Check sheet for the modelled part. Datum: model origin and axes. Units: mm. Face numbers are marked on the shaded views. A direction names the side the tool comes from. Give positions to 0.01 mm unless a question says otherwise; leave off trailing zeros. Write each loop counter-clockwise with the first axis right and the second up, starting at its lowest first coordinate (ties: lowest second). Pieces come first, ordered by that corner, then holes. Notation, with made-up numbers: (29.5, -31.75) -> (62.5, -31.75) arc R18 cw to (62.5, -1.75) -> close; hole circle Ø8 at (12, -15.75). An arc over 180 degrees is marked (long way). Answer as a JSON object with one key per item and string values.
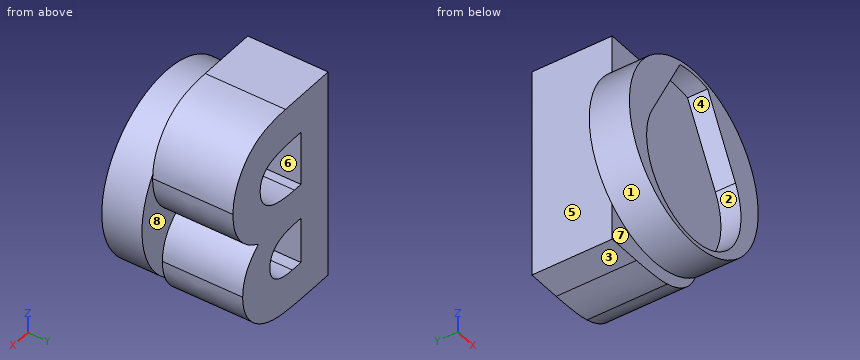
from build123d import *

# Parameters (mm, degrees)
SKETCH1_R           = 22.5
BOSS_EXTRUDE1_DEPTH = 10
BOSS_EXTRUDE2_DEPTH = 20
SKETCH3_R           = 16.5
CUT_EXTRUDE2_DEPTH  = 5


with BuildPart() as part:
    # Sketch1 → Boss-Extrude1 (new body)
    with BuildSketch(Plane(origin=(0, 0, 0), x_dir=(1, 0, 0), z_dir=(0, 1, 0))):
        with Locations(Location((0, 0, 0), (0, 0, 270))):
            Circle(SKETCH1_R)
    extrude(amount=BOSS_EXTRUDE1_DEPTH)

    # Sketch2 → Boss-Extrude2 (add)
    with BuildSketch(Plane(origin=(0, 10, 0), x_dir=(1, 0, 0), z_dir=(0, 1, 0))):
        with BuildLine():
            Line((-14.488149335, -26.70508671), (-14.488149335, 26.211579956))
            Line((-14.488149335, 26.211579956), (-6.007914293, 26.211579956))
            add(Edge.make_bspline(
                [(-6.007914293, 26.211579956), (-5.414244815, 26.211647709), (-4.265505631, 26.211778808), (-2.608174782, 26.15357879), (-1.071140386, 26.078290547), (0.340706119, 25.99406051), (1.629767793, 25.848915327), (2.794084408, 25.69594816), (3.835982274, 25.511479183), (4.480131109, 25.346004797), (4.783184799, 25.268153808)],
                knots=[0, 0, 0, 0, 1.311965854, 2.538629056, 3.664479157, 4.713267157, 5.663616078, 6.530575999, 7.308677837, 8, 8, 8, 8], degree=3))
            add(Edge.make_bspline(
                [(4.783184799, 25.268153808), (5.181125063, 25.158343602), (5.962011612, 24.942860725), (7.080490347, 24.507683744), (8.141523447, 24.023953675), (9.143815418, 23.472108139), (10.08121179, 22.845484813), (10.950150136, 22.139110625), (11.769371306, 21.381339407), (12.509786627, 20.551052288), (13.179000085, 19.673700144), (13.760426595, 18.749512867), (14.265611712, 17.792621882), (14.669892129, 16.790985354), (14.974509828, 15.749216088), (15.197305942, 14.671762602), (15.341707994, 13.555215567), (15.355352093, 12.795592125), (15.362278015, 12.409997424)],
                knots=[0, 0, 0, 0, 1.099996261, 2.158545794, 3.195537121, 4.207578794, 5.205712374, 6.197378256, 7.190519799, 8.17788031, 9.159561366, 10.129234751, 11.085776129, 12.040971148, 13.00380137, 13.975669004, 14.972423361, 16, 16, 16, 16], degree=3))
            add(Edge.make_bspline(
                [(15.362278015, 12.409997424), (15.344168787, 11.914609447), (15.308522997, 10.939499081), (15.080815259, 9.507238371), (14.653827774, 8.153546136), (14.095125035, 6.85347434), (13.335463983, 5.611872259), (12.370841368, 4.429330241), (11.216880916, 3.269436044), (10.331729546, 2.574157712), (9.871325825, 2.212514786)],
                knots=[0, 0, 0, 0, 0.986156485, 1.941127874, 2.875419072, 3.804401753, 4.751181392, 5.761612777, 6.835722519, 8, 8, 8, 8], degree=3))
            add(Edge.make_bspline(
                [(9.871325825, 2.212514786), (10.244414913, 2.022056041), (10.975939394, 1.648619138), (12.014489248, 1.034800345), (12.976073045, 0.381926211), (13.865002238, -0.296867174), (14.662630517, -1.030354847), (15.401893295, -1.77627224), (16.046319182, -2.577357317), (16.622584233, -3.40505788), (17.123464449, -4.271359131), (17.559675885, -5.174798081), (17.928128038, -6.118461074), (18.240142851, -7.09754563), (18.472843581, -8.115419342), (18.624569406, -9.172446243), (18.740740181, -10.265021335), (18.749777175, -11.009256203), (18.754372032, -11.387662164)],
                knots=[0, 0, 0, 0, 1.164658916, 2.283573913, 3.35186032, 4.395461096, 5.390182219, 6.362969632, 7.312859996, 8.245001507, 9.165155236, 10.092416118, 11.032087915, 11.979892451, 12.947605196, 13.931445124, 14.948243989, 16, 16, 16, 16], degree=3))
            add(Edge.make_bspline(
                [(18.754372032, -11.387662164), (18.724554483, -12.110395914), (18.665709669, -13.536708072), (18.235465105, -15.630861893), (17.48955774, -17.616309656), (16.487957959, -19.48516034), (15.25379432, -21.183313786), (13.834860053, -22.670881463), (12.245440572, -23.930074476), (10.779008994, -24.779932076), (9.510661162, -25.350265997), (8.46011235, -25.702882393), (7.331845194, -26.029545689), (6.105192549, -26.258935401), (4.802391955, -26.468898089), (3.410741024, -26.598533402), (1.932840727, -26.686384059), (0.917754918, -26.698726455), (0.394663165, -26.70508671)],
                knots=[0, 0, 0, 0, 1.284142165, 2.534249414, 3.780121997, 5.041676246, 6.291546858, 7.49970053, 8.684500223, 9.883330709, 10.50184324, 11.153274765, 11.851151195, 12.587658647, 13.369265475, 14.195992086, 15.070362669, 16, 16, 16, 16], degree=3))
            Line((0.394663165, -26.70508671), (-14.488149335, -26.70508671))
        make_face()
        with BuildLine():
            Line((-4.990286087, 16.713716709), (-4.990286087, 5.180597051))
            Line((-4.990286087, 5.180597051), (-2.467416162, 5.180597051))
            add(Edge.make_bspline(
                [(-2.467416162, 5.180597051), (-2.124535473, 5.1835871), (-1.462625052, 5.189359209), (-0.50656566, 5.263701973), (0.382415177, 5.390535346), (1.200945746, 5.567499807), (1.956650957, 5.79221887), (2.644703146, 6.062604299), (3.262077073, 6.392503912), (3.979322786, 6.883903943), (4.737503228, 7.607021089), (5.404920943, 8.65171363), (5.798025521, 9.853106078), (5.841806769, 10.700421057), (5.864414767, 11.137962168)],
                knots=[0, 0, 0, 0, 1.065314748, 2.056525647, 2.977365736, 3.853934255, 4.656397591, 5.425096493, 6.14721249, 6.826394842, 8.123232004, 9.372140726, 10.643011755, 12, 12, 12, 12], degree=3))
            add(Edge.make_bspline(
                [(5.864414767, 11.137962168), (5.84632423, 11.547792116), (5.811346902, 12.340181849), (5.415541135, 13.452767604), (4.800776528, 14.438746288), (4.074960502, 15.113568064), (3.391463676, 15.574451442), (2.80621175, 15.87792352), (2.163853815, 16.149588622), (1.451954509, 16.357310381), (0.674579167, 16.513177474), (-0.164496065, 16.627643188), (-1.06671888, 16.705553423), (-1.689886099, 16.710937246), (-2.011603529, 16.713716709)],
                knots=[0, 0, 0, 0, 1.347982417, 2.606269829, 3.849316587, 5.153353503, 5.842674298, 6.568177932, 7.326619318, 8.142485038, 9.012069166, 9.942760135, 10.937925643, 12, 12, 12, 12], degree=3))
            Line((-2.011603529, 16.713716709), (-4.990286087, 16.713716709))
        make_face(mode=Mode.SUBTRACT)
        with BuildLine():
            Line((-4.990286087, -3.638847394), (-4.990286087, -17.207223462))
            Line((-4.990286087, -17.207223462), (-2.255410286, -17.207223462))
            add(Edge.make_bspline(
                [(-2.255410286, -17.207223462), (-1.714721858, -17.204134529), (-0.675180886, -17.198195671), (0.813959715, -17.126440131), (2.167960807, -16.997113416), (3.383234797, -16.835659429), (4.461643108, -16.61691453), (5.399540462, -16.338808424), (6.209788904, -16.032843269), (6.887530146, -15.654939974), (7.441205914, -15.215154252), (7.940840245, -14.76568268), (8.348210945, -14.247174757), (8.670530245, -13.681888592), (8.94949703, -13.0838663), (9.117750095, -12.429755326), (9.245852073, -11.738941952), (9.252901868, -11.26112128), (9.256508784, -11.016651881)],
                knots=[0, 0, 0, 0, 1.753078804, 3.370512758, 4.83203934, 6.162291463, 7.344201807, 8.395507345, 9.331626367, 10.147333109, 10.898971645, 11.62040215, 12.321813352, 13.025280112, 13.727906689, 14.453419512, 15.208716525, 16, 16, 16, 16], degree=3))
            add(Edge.make_bspline(
                [(9.256508784, -11.016651881), (9.248554499, -10.737097279), (9.233061691, -10.192600118), (9.106531742, -9.396759406), (8.876585491, -8.653789298), (8.58695697, -7.944691045), (8.183923494, -7.294852835), (7.704931981, -6.681786232), (7.126187955, -6.126251562), (6.475356533, -5.594648013), (5.716226117, -5.129200305), (4.848440543, -4.725341973), (3.867285527, -4.388054368), (2.769721839, -4.119505755), (1.560561113, -3.891592259), (0.230977803, -3.755502742), (-1.207954859, -3.654286988), (-2.205734185, -3.644110867), (-2.721823214, -3.638847394)],
                knots=[0, 0, 0, 0, 0.845221588, 1.646264278, 2.427170338, 3.19324141, 3.95557735, 4.731569926, 5.540061037, 6.376114724, 7.268642756, 8.224665384, 9.265483498, 10.400594375, 11.639216012, 12.983232105, 14.439614077, 16, 16, 16, 16], degree=3))
            Line((-2.721823214, -3.638847394), (-4.990286087, -3.638847394))
        make_face(mode=Mode.SUBTRACT)
    extrude(amount=BOSS_EXTRUDE2_DEPTH)

    # Sketch3 → Cut-Extrude2 (cut)
    with BuildSketch(Plane.XZ):
        with BuildLine():
            ThreePointArc((-14.551420086, 2.778571429), (0, 11.5), (14.551420086, 2.778571429))
            Line((14.551420086, 2.778571429), (4.83856504, 20.948467447))
            ThreePointArc((4.83856504, 20.948467447), (0, 21.5), (-4.83856504, 20.948467447))
            Line((-4.83856504, 20.948467447), (-14.551420086, 2.778571429))
        make_face()
        with Locations((0, -5)):
            Circle(SKETCH3_R)
    extrude(amount=-CUT_EXTRUDE2_DEPTH, mode=Mode.SUBTRACT)


solid = part.part
1. Sectioned sample at B-B, the plane y = 19. State how many separate pieces and enclosed holes the cut face has, plus the area to 3 significant figures.
Determined:
{"separate pieces": "1", "enclosed holes": "2", "area": "1,250 mm^2"}
2. Sectioned sample at D-D, the plane x = 20. Enter the section's corners in (y, z), plus the area to 3 significant figures.
Determined:
{"outline": "(0, -10.31) -> (10, -10.31) -> (10, 10.31) -> (0, 10.31) -> close", "area": "206 mm^2"}
3. Sectioned sample at C-C, the plane x = -19. Enter the section's corners in (y, z), plus the area to 3 significant figures.
Determined:
{"outline": "(0, -12.05) -> (10, -12.05) -> (10, 12.05) -> (0, 12.05) -> close", "area": "241 mm^2"}
4. Mould release check, pull along Z, two halves, no side actions. Record for the marked faces 1, 2 and 3: released by +Z, released by -Z, zero draft, split by the parting line, or undercut.
Determined:
{"face 1": "split by the parting line", "face 2": "undercut", "face 3": "released by -Z"}
5. Access from +Z, -Z, +X, -X, +Y, -Y to the whole of each face (thin tool, end or side, straight path). Record for the marked faces 4, 5, 6, 7 and 8.
Determined:
{"face 4": "-Y", "face 5": "+Z, -Z, -X, +Y", "face 6": "+Y", "face 7": "-Z, -Y", "face 8": "+X, +Y"}
6. Sectioned sample at A-A, the plane y = 2.5. Enter the section's corners in (x, z), plus the area to 3 significant figures.
Determined:
{"outline": "circle Ø45 at (0, 0); hole (-14.55, 2.78) arc R16.5 ccw (long way) to (14.55, 2.78) -> (4.84, 20.95) arc R21.5 ccw to (-4.84, 20.95) -> close", "area": "560 mm^2"}
7. Go/stop test with flat-tipped pins: P1, Ø8.5, axis at x = 0, z = -12, coming from the +Y side; P2, Ø6, axis at y = 4.5, z = 10.5, coming from the +X side; P3, Ø12.5, axis at y = 20, z = -11, coming from the +X side. Record where each tip stops, or that it passes through.
Determined:
{"P1": "y = 10", "P2": "x = 21.21", "P3": "x = 15.36"}
8. Scan lines: L1, parallel to Z at x = -2.5, y = 13; L2, parallel to Y at x = 15, z = 1.5; L3, parallel to X at y = 17, z = 14. Record each from-to range of solid material in increasing order. Write a range as [from, to].
Determined:
{"L1": "[-26.15, -16.71], [-5.18, 3.64], [17.21, 26.71]", "L2": "[5, 30]", "L3": "[-14.49, -4.99], [8.48, 18.54]"}
